Build history of the part. All positions in model axes, mm. Give positions to 0.01 mm unless a question says otherwise; leave off trailing zeros. Order: outer loops, then holes, each group sorted by start corner. A loop starts at its lowest first (then second) coordinate and runs counter-clockwise, first axis right, second up. Notation, with made-up numbers: (10.25, 7.25) -> (52.25, 7.25) arc R13 cw to (52.25, 18.25) -> close; hole circle Ø8 at (-24, 37). An arc over 180 degrees is marked (long way). Write item = value, one per line. Start each with the question number.
from build123d import *

# Parameters (mm, degrees)
F0_R      = 24.946026
F1_DEPTH  = 75.1
F2_R      = 9.571884
F2_R_2    = 24.946026
F1_FACE_R = 24.946026
F3_DEPTH  = 85
F4_R      = 9.504861
F5_DEPTH  = 84.9
F6_R      = 9.521751
F7_DEPTH  = 84.7
F8_R      = 9.589017
F9_DEPTH  = 94.3


with BuildPart() as f1:
    # F0 (on Top) → F1 (new body)
    with BuildSketch(Plane.XY):
        Circle(F0_R)
    extrude(amount=F1_DEPTH)

    # F2 (on face) + F1_face (on face) → F3 (join)
    with BuildSketch(Plane(origin=(0, 0, 0), x_dir=(1, 0, 0), z_dir=(0, 0, -1))):
        Circle(F2_R)
        Circle(F2_R_2)
        Circle(F2_R, mode=Mode.SUBTRACT)
    with BuildSketch(Plane(origin=(0, 0, 0), x_dir=(1, 0, 0), z_dir=(0, 0, -1))):
        Circle(F1_FACE_R)
    extrude(amount=-F3_DEPTH)

    # F4 (on face) → F5 (join)
    with BuildSketch(Plane.XY.offset(85)):
        Circle(F4_R)
    extrude(amount=-F5_DEPTH)

    # F6 (on face) → F7 (join)
    with BuildSketch(Plane(origin=(0, 0, 0), x_dir=(1, 0, 0), z_dir=(0, 0, -1))):
        Circle(F6_R)
    extrude(amount=-F7_DEPTH)

    # F8 (on Top) → F9 (cut)
    with BuildSketch(Plane.XY):
        Circle(F8_R)
    extrude(amount=F9_DEPTH, mode=Mode.SUBTRACT)


solid = f1.part
(1) Wall check: line 1 (X direction, y = 0, z = 47); line 2 (Y direction, x = 3.5, z = 36.5). Give the ranges that are in metal, low to high. Write a range as [from, to].
(2) Mould opens along X. For faces 1 (the face through (0, -11, 0)), 2 (the face through (-1.248, 9.507, 41.905)), 3 (the face through (-3.247, 24.734, 41.905)) say: released by +X, released by -X, zero draft, split by the parting line, or undercut.
(3) Cut at C-C, the plane z = 76.5. Give the cut face in (x, y).
(4) Cut at D-D, the plane y = 19. Give the cut face in (x, z).
(5) Cut at A-A, the plane x = 0. Give the cut face in (y, z), plus the area to 3 significant figures.
(6) Flat gauge pins, fed straight in: P1, Ø5, axis at y = 15, z = 28, coming from the -X side; P2, Ø11.5, axis at x = 0, y = 0, coming from the +Z side; P3, Ø6, axis at x = -3.5, z = 45, coming from the -Y side; P4, Ø6, axis at y = -9.5, z = 55.5, coming from the +X side. Where does each tip first touch, or does it go through?
Results:
q1.line_1 = [-24.95, -9.59], [9.59, 24.95]
q1.line_2 = [-24.7, -8.93], [8.93, 24.7]
q2.face_1 = zero draft
q2.face_2 = undercut
q2.face_3 = split by the parting line
q3.outline = circle Ø49.89 at (0, 0); hole circle Ø19.18 at (0, 0)
q4.outline = (-16.16, 0) -> (16.16, 0) -> (16.16, 85) -> (-16.16, 85) -> close
q5.outline = (-24.95, 0) -> (-9.59, 0) -> (-9.59, 85) -> (-24.95, 85) -> close; (9.59, 0) -> (24.95, 0) -> (24.95, 85) -> (9.59, 85) -> close
q5.area = 2,610 mm2
q6.P1 = -21.59
q6.P2 = through
q6.P3 = -24.94
q6.P4 = 24.08
